CAD build for the part. Positions are in the model's coordinates, mm. Give positions to 0.01 mm unless a question says otherwise; leave off trailing zeros. Order: outer loops, then holes, each group sorted by start corner. A loop starts at its lowest first (then second) coordinate and runs counter-clockwise, first axis right, second up.
Item 1: Wall check: L1, parallel to Y at x = 102.5, z = 1.45; L2, parallel to X at y = -4.5, z = 0.6; L3, parallel to Y at x = -45.5, z = 0.85. Give the ranges that are in metal, low to high.
Item 2: Band-saw the part on C-C on z = 0.8. Count the separate pieces of the cut face and the enclosed holes in it, plus the area to 3 significant figures.
Item 3: Band-saw the part on A-A on x = -13. Give the cut face in (y, z), plus the area to 3 significant figures.
Item 4: Flat gauge pin, fed straight in: P1, Ø1.6, axis at x = -86.5, y = 42, coming from the -Z side. Where does the tip first touch, or does it go through?
Item 5: Two-plate mould, pull along X, no slides. Class faces 1 (the flat face through (-2, 1, 2)), 2 (the cylindrical face through (-49.5, 14, 1)): released by +X, released by -X, zero draft, split by the parting line, or undercut.
Item 6: Band-saw the part on B-B on x = 67.5. Give the cut face in (y, z).
```python
from build123d import *

# Parameters (mm, degrees)
SKETCH_1_W                  = 215
SKETCH_1_H                  = 110
SKETCH_1_R                  = 2.25
SKETCH_1_R_2                = 5
EXTRUDE_1_DEPTH             = 2
SKETCH_3_R                  = 0.55
CUT_EXTRUDE_1_DEPTH         = 2
PATTERN_LINEAR_1_COUNT      = 2
PATTERN_LINEAR_1_PITCH      = 2
PATTERN_LINEAR_1_COUNT_DIR2 = 12
PATTERN_LINEAR_1_PITCH_DIR2 = 2.54
SKETCH_4_R                  = 0.9
SKETCH_4_R_2                = 0.8
CUT_EXTRUDE_2_DEPTH         = 2


with BuildPart() as part:
    # Эскиз1 → Вытянуть1 (new body)
    with BuildSketch(Plane.XY):
        Rectangle(SKETCH_1_W, SKETCH_1_H)
        with Locations((-102.5, 42)):
            Circle(SKETCH_1_R, mode=Mode.SUBTRACT)
        with Locations((102.5, 42)):
            Circle(SKETCH_1_R, mode=Mode.SUBTRACT)
        with Locations((102.5, -42)):
            Circle(SKETCH_1_R, mode=Mode.SUBTRACT)
        with Locations((-102.5, -42)):
            Circle(SKETCH_1_R, mode=Mode.SUBTRACT)
        with Locations((-45.5, 17)):
            Circle(SKETCH_1_R_2, mode=Mode.SUBTRACT)
        with Locations((-13, 17)):
            Circle(SKETCH_1_R_2, mode=Mode.SUBTRACT)
        with Locations((-13, -17)):
            Circle(SKETCH_1_R_2, mode=Mode.SUBTRACT)
        with Locations((-45.5, -17)):
            Circle(SKETCH_1_R_2, mode=Mode.SUBTRACT)
        with Locations((52.5, -37)):
            Circle(SKETCH_1_R_2, mode=Mode.SUBTRACT)
        with Locations((67.5, 15)):
            Circle(SKETCH_1_R, mode=Mode.SUBTRACT)
    extrude(amount=EXTRUDE_1_DEPTH)

    # Эскиз3 → Вырез-Вытянуть1 (cut)
    with BuildSketch(Plane.XY.offset(2)):
        with Locations((1.5, 15.72)):
            Circle(SKETCH_3_R)
    cut_extrude_1 = extrude(amount=-CUT_EXTRUDE_1_DEPTH, mode=Mode.SUBTRACT)

    # Линейный массив1: Cut-Extrude 1 2 × 12
    with Locations(*[(i * PATTERN_LINEAR_1_PITCH, -j * PATTERN_LINEAR_1_PITCH_DIR2, 0) for i in range(PATTERN_LINEAR_1_COUNT) for j in range(PATTERN_LINEAR_1_COUNT_DIR2) if (i, j) != (0, 0)]):
        add(cut_extrude_1, mode=Mode.SUBTRACT)

    # Эскиз4 → Вырез-Вытянуть2 (cut)
    with BuildSketch(Plane.XY.offset(2)):
        with Locations((15.5, 49.4)):
            Circle(SKETCH_4_R)
        with Locations((15.5, 44.32)):
            Circle(SKETCH_4_R)
        with Locations((15.5, 39.24)):
            Circle(SKETCH_4_R)
        with Locations((15.5, 34.16)):
            Circle(SKETCH_4_R)
        with Locations((15.5, 29.08)):
            Circle(SKETCH_4_R)
        with Locations((15.5, -16)):
            Circle(SKETCH_4_R)
        with Locations((15.5, 9.16)):
            Circle(SKETCH_4_R)
        with Locations((15.5, 4.08)):
            Circle(SKETCH_4_R)
        with Locations((15.5, -1)):
            Circle(SKETCH_4_R)
        with Locations((15.5, -31.24)):
            Circle(SKETCH_4_R)
        with Locations((15.5, -21.08)):
            Circle(SKETCH_4_R)
        with Locations((15.5, -26.16)):
            Circle(SKETCH_4_R)
        with Locations((-86.5, 42)):
            Circle(SKETCH_4_R)
        with Locations((-81.42, 42)):
            Circle(SKETCH_4_R)
        with Locations((10.5, -43.5)):
            Circle(SKETCH_4_R_2)
        with Locations((15.5, -43.5)):
            Circle(SKETCH_4_R_2)
        with Locations((20.5, -43.5)):
            Circle(SKETCH_4_R_2)
        with Locations((25.5, -43.5)):
            Circle(SKETCH_4_R_2)
        with Locations((30.5, -43.5)):
            Circle(SKETCH_4_R_2)
    extrude(amount=-CUT_EXTRUDE_2_DEPTH, mode=Mode.SUBTRACT)


solid = part.part
```
The answers:
1. L1: y = -55 to -44.25, -39.75 to 39.75, 44.25 to 55
1. L2: x = -107.5 to 0.96, 2.04 to 2.96, 4.04 to 107.5
1. L3: y = -55 to -22, -12 to 12, 22 to 55
2. separate pieces: 1
2. enclosed holes: 53
2. area: 23,100 mm2
3. outline: (-55, 0) - (-22, 0) - (-22, 2) - (-55, 2) - close; (-12, 0) - (12, 0) - (12, 2) - (-12, 2) - close; (22, 0) - (55, 0) - (55, 2) - (22, 2) - close
3. area: 180 mm2
4. P1: passes through
5. face 1: zero draft
5. face 2: undercut
6. outline: (-55, 0) - (12.75, 0) - (12.75, 2) - (-55, 2) - close; (17.25, 0) - (55, 0) - (55, 2) - (17.25, 2) - close
